Read the model definition and answer for the solid it produces. Units are mm, in the model's axes. A direction names the side the tool comes from. Round coordinates to 2 decimals unless told otherwise and drop trailing zeros. Order: outer loops, then holes, each group sorted by start corner. A loop starts at its lowest first (then second) coordinate and runs counter-clockwise, first axis right, second up. Notation, with made-up numbers: (72, -37) - (115, -37) arc R12 cw to (115, -17) - close; hole circle Ø10 at (2.25, -14). An arc over 180 degrees is marked (long way). Answer as a JSON object with one key per item and string values. Group by question number.
Q1. A cutting plane is placed at C-C on z = 22. Determine the outline of the cut face in (x, y), and give its area (3 significant figures).
Q2. A cutting plane is placed at B-B on x = 8.75. Determine the outline of the cut face in (y, z), and give its area (3 significant figures).
Q3. The mould has two halves that part along Z. Classify faces 5 (the cylindrical face through (13.199, 8.112, 7.215)), 6 (the flat face through (0, 0, 6)), 7 (the cylindrical face through (6.243, 9.098, -11.198)): pulls with the +Z half, pulls with the -Z half, needs draft (parallel to the pull), parting line crosses it, or undercut.
Q4. A cutting plane is placed at A-A on z = -10. Determine the outline of the cut face in (x, y) (3 decimals).
Q5. Given pin 1 Ø14 at (x, z) = (4, -0.5) entering from -Y; pin 2 Ø3 at (x, z) = (0, 18.5) entering from -Y; pin 3 Ø2.5 at (y, z) = (7, -10.5) entering from -X; pin 4 Ø6.5 at (y, z) = (6.5, -4) entering from -X, each flat-ended and moving along its own axis, determine where each tip first touches the part or whether it passes through.
Q6. A cutting plane is placed at D-D on y = 8.75. Count the separate pieces of the cut face and the enclosed holes in it, and give its area (3 significant figures).
Q7. A tool of negligible diameter and unlimited length cuts with its end or side. For faces 1 (the cylindrical face through (-7.834, 0.301, 7.215)), 2 (the flat face through (-6, 3, -10)), 3 (the flat face through (-1.727, 8.021, 16.813)), 4 (the cylindrical face through (2.21, 9.17, 23.11)), from which of +Z, -Z, +X, -X, +Y, -Y can it reach the whole face along a straight path? Write none if from no direction.
Q8. Consider line 1 (Y direction, x = 6.3, z = -10) (3 decimals); line 2 (X direction, y = 4.75, z = -9.5); line 3 (Y direction, x = 10.75, z = -5.5). Determine where each line is inside the solid, lowest interval first.
```python
from build123d import *

# Parameters (mm, degrees)
ESQUISSE1_W             = 27
ESQUISSE1_H             = 15
BOSS_EXTRU_1_DEPTH      = 16
ESQUISSE2_W             = 1
ESQUISSE2_H             = 12.860678648
ENL_V_MAT_EXTRU_1_DEPTH = 16
ESQUISSE3_W             = 12.860678648
ESQUISSE3_H             = 1
ENL_V_MAT_EXTRU_2_DEPTH = 26
ESQUISSE4_R             = 6.375627484
BOSS_EXTRU_2_DEPTH      = 3
ESQUISSE5_R             = 2.5
BOSS_EXTRU_3_DEPTH      = 15
CONG_4_R                = 1
ESQUISSE6_W             = 7.518022456
ESQUISSE6_H             = 15.453712828
ENL_V_MAT_EXTRU_4_DEPTH = 6.5
ESQUISSE7_W             = 7.269073366
ESQUISSE7_H             = 15.09730622
ENL_V_MAT_EXTRU_5_DEPTH = 6.5
ENL_V_MAT_EXTRU_6_DEPTH = 6.5
CONG_5_R                = 1
CONG_6_R                = 1
ESQUISSE9_W             = 1
ESQUISSE9_H             = 10
BOSS_EXTRU_4_DEPTH      = 5
ESQUISSE10_R            = 1.625
ENL_V_MAT_EXTRU_7_DEPTH = 18


with BuildPart() as part:
    # Esquisse1 → Boss.-Extru.1 (new body)
    with BuildSketch(Plane(origin=(0, 0, 0), x_dir=(1, 0, 0), z_dir=(0, 1, 0))):
        Rectangle(ESQUISSE1_W, ESQUISSE1_H)
    extrude(amount=BOSS_EXTRU_1_DEPTH)

    # Esquisse2 → Enlèv. mat.-Extru.1 (cut)
    with BuildSketch(Plane.XZ):
        with Locations((-13, -1.069660676)):
            Rectangle(ESQUISSE2_W, ESQUISSE2_H)
        with Locations((13, -1.069660676)):
            Rectangle(ESQUISSE2_W, ESQUISSE2_H)
    extrude(amount=-ENL_V_MAT_EXTRU_1_DEPTH, mode=Mode.SUBTRACT)

    # Esquisse3 → Enlèv. mat.-Extru.2 (cut)
    with BuildSketch(Plane(origin=(12.5, 0, 0), x_dir=(0, 0, -1), z_dir=(1, 0, 0))):
        with Locations((1.069660676, 0.5)):
            Rectangle(ESQUISSE3_W, ESQUISSE3_H)
        with Locations((1.069660676, 15.5)):
            Rectangle(ESQUISSE3_W, ESQUISSE3_H)
    extrude(amount=-ENL_V_MAT_EXTRU_2_DEPTH, mode=Mode.SUBTRACT)

    # Esquisse4 → Boss.-Extru.2 (add)
    with BuildSketch(Plane.XY.offset(7.5)):
        with Locations((0, 8)):
            Circle(ESQUISSE4_R)
    extrude(amount=BOSS_EXTRU_2_DEPTH)

    # Esquisse5 → Boss.-Extru.3 (add)
    with BuildSketch(Plane.XY.offset(10.5)):
        with Locations((0, 8)):
            Circle(ESQUISSE5_R)
    extrude(amount=BOSS_EXTRU_3_DEPTH)

    # Congé4
    cong_4_edges = [part.edges().sort_by_distance(p)[0] for p in [
        (-2.5, 8, 25.5),
    ]]
    fillet(cong_4_edges, radius=CONG_4_R)

    # Esquisse6 → Enlèv. mat.-Extru.4 (cut)
    with BuildSketch(Plane(origin=(0, 16, 0), x_dir=(1, 0, 0), z_dir=(0, 1, 0))):
        with Locations((0, -18.226856414)):
            Rectangle(ESQUISSE6_W, ESQUISSE6_H)
    extrude(amount=-ENL_V_MAT_EXTRU_4_DEPTH, mode=Mode.SUBTRACT)

    # Esquisse7 → Enlèv. mat.-Extru.5 (cut)
    with BuildSketch(Plane.XZ):
        with Locations((0, 18.04865311)):
            Rectangle(ESQUISSE7_W, ESQUISSE7_H)
    extrude(amount=-ENL_V_MAT_EXTRU_5_DEPTH, mode=Mode.SUBTRACT)

    # Esquisse8 → Enlèv. mat.-Extru.6 (cut)
    with BuildSketch(Plane(origin=(0, 9.5, 0), x_dir=(1, 0, 0), z_dir=(0, 1, 0))):
        Polygon((2, -19.525589234), (2, -10.5), (0.951197678, -10.5), (0.951197678, -12.063973085), (1.25, -12.063973085), align=None)
        Polygon((2.5, -24.5), (2.5, -10.5), (2, -10.5), (2, -19.525589234), align=None)
        Polygon((-2.5, -10.5), (-0.951197678, -10.5), (-0.951197678, -12.063973085), (-1.25, -12.063973085), (-2.5, -24.5), align=None)
    extrude(amount=-ENL_V_MAT_EXTRU_6_DEPTH, mode=Mode.SUBTRACT)

    # Congé5
    cong_5_edges = [part.edges().sort_by_distance(p)[0] for p in [
        (-6.375627484, 8, 7.5),
        (-6.375627484, 8, 10.5),
    ]]
    fillet(cong_5_edges, radius=CONG_5_R)

    # Congé6
    cong_6_edges = [part.edges().sort_by_distance(p)[0] for p in [
        (0, 16, 7.5),
        (0, 0, 7.5),
        (13.5, 8, 7.5),
        (-13.5, 8, 7.5),
    ]]
    fillet(cong_6_edges, radius=CONG_6_R)

    # Esquisse9 → Boss.-Extru.4 (add)
    with BuildSketch(Plane(origin=(0, 0, -7.5), x_dir=(-1, 0, 0), z_dir=(0, 0, -1))):
        with Locations((6.25, 8)):
            Rectangle(ESQUISSE9_W, ESQUISSE9_H)
        with Locations((-6.25, 8)):
            Rectangle(ESQUISSE9_W, ESQUISSE9_H)
    extrude(amount=BOSS_EXTRU_4_DEPTH)

    # Esquisse10 → Enlèv. mat.-Extru.7 (cut)
    with BuildSketch(Plane.ZY.offset(6.75)):
        with Locations((-10, 8)):
            Circle(ESQUISSE10_R)
    extrude(amount=-ENL_V_MAT_EXTRU_7_DEPTH, mode=Mode.SUBTRACT)


solid = part.part
```
Result set:
{
 "1": {"outline": "(-2.25, 6.91) arc R2.5 ccw to (-2, 6.5) - (2, 6.5) arc R2.5 ccw to (2.25, 6.91) - (2.25, 9.09) arc R2.5 ccw to (2, 9.5) - (-2, 9.5) arc R2.5 ccw to (-2.25, 9.09) - close", "area": "13.3 mm²"},
 "2": {"outline": "(0, 5.36) - (1, 5.36) - (1, -7.5) - (15, -7.5) - (15, 5.36) - (16, 5.36) - (16, 6.5) arc R1 ccw to (15, 7.5) - (1, 7.5) arc R1 ccw to (0, 6.5) - close", "area": "214 mm²"},
 "3": {"face 5": "pulls with the +Z half", "face 6": "needs draft", "face 7": "undercut"},
 "4": {"outline": "(-6.75, 3) - (-5.75, 3) - (-5.75, 6.375) - (-6.75, 6.375) - close; (-6.75, 9.625) - (-5.75, 9.625) - (-5.75, 13) - (-6.75, 13) - close; (5.75, 3) - (6.75, 3) - (6.75, 6.375) - (5.75, 6.375) - close; (5.75, 9.625) - (6.75, 9.625) - (6.75, 13) - (5.75, 13) - close"},
 "5": {"pin 1": "stops at y = 0", "pin 2": "stops at y = 6.5", "pin 3": "stops at x = -6.75", "pin 4": "stops at x = -12.5"},
 "6": {"separate pieces": "3", "enclosed holes": "0", "area": "475 mm²"},
 "7": {"face 1": "+Z, -X, -Y", "face 2": "-Z, +X, -X, -Y", "face 3": "-X, +Y, -Y", "face 4": "+Z, +X, +Y"},
 "8": {"line 1": "y = 3 to 6.375, 9.625 to 13", "line 2": "x = -6.75 to -5.75, 5.75 to 6.75", "line 3": "y = 1 to 15"}
}
